```python
from build123d import *

# Parameters (mm, degrees)
ESQUISSE1_W             = 19.5
ESQUISSE1_H             = 1.5
EXTRU_MINCE1_DEPTH      = 127.5
ESQUISSE2_W             = 1.5
ESQUISSE2_H             = 19.5
EXTRU_MINCE2_DEPTH      = 255
ENL_V_MAT_EXTRU_1_DEPTH = 130.132925701
ESQUISSE4_R             = 2.5
ENL_V_MAT_EXTRU_2_DEPTH = 130.409234601
ESQUISSE5_R             = 1.5
ENL_V_MAT_EXTRU_3_DEPTH = 130.350541166
ESQUISSE6_R             = 1.5
ENL_V_MAT_EXTRU_4_DEPTH = 130.409234601


with BuildPart() as part:
    # Esquisse1 → Extru.-Mince1 (new, symmetric)
    with BuildSketch(Plane.XY):
        with Locations((0, 0.75)):
            Rectangle(ESQUISSE1_W, ESQUISSE1_H)
    extrude(amount=EXTRU_MINCE1_DEPTH, both=True)

    # Esquisse2 → Extru.-Mince2 (add)
    with BuildSketch(Plane(origin=(0, 0, -127.5), x_dir=(-1, 0, 0), z_dir=(0, 0, -1))):
        with Locations((0, 9.75)):
            Rectangle(ESQUISSE2_W, ESQUISSE2_H)
    extrude(amount=-EXTRU_MINCE2_DEPTH)

    # Esquisse3 → Enlèv. mat.-Extru.1 (cut, through all)
    with BuildSketch(Plane(origin=(0, 1.5, 0), x_dir=(1, 0, 0), z_dir=(0, 1, 0))):
        with BuildLine():
            Line((-0.75, 127.5), (-0.75, 110))
            ThreePointArc((-0.75, 110), (-8.75, 102), (-16.75, 110))
            Line((-16.75, 110), (-16.75, 127.5))
            ThreePointArc((-16.75, 127.5), (-8.75, 135.5), (-0.75, 127.5))
        make_face()
        with BuildLine():
            Line((17.75, 10), (17.75, -10))
            ThreePointArc((17.75, -10), (9.75, -18), (1.75, -10))
            Line((1.75, -10), (1.75, 10))
            ThreePointArc((1.75, 10), (9.75, 18), (17.75, 10))
        make_face()
        with BuildLine():
            Line((-16.75, -127.5), (-16.75, -110))
            ThreePointArc((-16.75, -110), (-8.75, -102), (-0.75, -110))
            Line((-0.75, -110), (-0.75, -127.5))
            ThreePointArc((-0.75, -127.5), (-8.75, -135.5), (-16.75, -127.5))
        make_face()
    extrude(amount=-ENL_V_MAT_EXTRU_1_DEPTH, mode=Mode.SUBTRACT)

    # Esquisse4 → Enlèv. mat.-Extru.2 (cut, through all)
    with BuildSketch(Plane(origin=(0.75, 0, 0), x_dir=(0, 0, -1), z_dir=(1, 0, 0))):
        with Locations((-120, 10.5)):
            Circle(ESQUISSE4_R)
        with Locations((120, 10.5)):
            Circle(ESQUISSE4_R)
    extrude(amount=-ENL_V_MAT_EXTRU_2_DEPTH, mode=Mode.SUBTRACT)

    # Esquisse5 → Enlèv. mat.-Extru.3 (cut, through all)
    with BuildSketch(Plane.XZ):
        with Locations(Location((-5.75, 59, 0), (0, 0, 270))):
            Circle(ESQUISSE5_R)
        with Locations(Location((-5.75, -59, 0), (0, 0, 90))):
            Circle(ESQUISSE5_R)
    extrude(amount=-ENL_V_MAT_EXTRU_3_DEPTH, mode=Mode.SUBTRACT)

    # Esquisse6 → Enlèv. mat.-Extru.4 (cut, through all)
    with BuildSketch(Plane(origin=(0.75, 0, 0), x_dir=(0, 0, -1), z_dir=(1, 0, 0))):
        with Locations((-51, 6.5)):
            Circle(ESQUISSE6_R)
        with Locations((-15, 6.5)):
            Circle(ESQUISSE6_R)
        with Locations((15, 6.5)):
            Circle(ESQUISSE6_R)
        with Locations((51, 6.5)):
            Circle(ESQUISSE6_R)
    extrude(amount=-ENL_V_MAT_EXTRU_4_DEPTH, mode=Mode.SUBTRACT)


solid = part.part
```
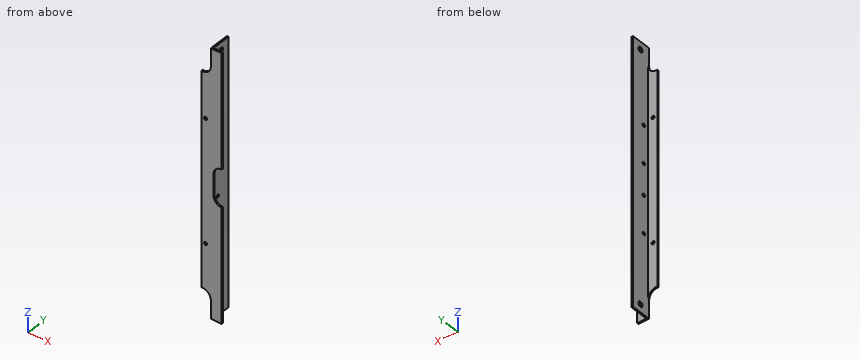
Geometry: final body of the model. Coordinates: model frame, mm. Coordinates: 2 decimals unless noted, no trailing zeros. Order: outer loops, then holes, each group sorted by start corner. A loop starts at its lowest first (then second) coordinate and runs counter-clockwise, first axis right, second up. Notation, with made-up numbers: (38.25, 8.25) - (66.25, 8.25) arc R13 ccw to (66.25, 21.25) - close; hole circle Ø6 at (-25.5, -7). An arc over 180 degrees is marked (long way). Write each question's results on one line, items separated by ' | '.
1) Section C-C, the plane x = 5.25. Return loops of the section in (y, z), plus the area to 3 significant figures.
Results list:
outline: (0, -127.5) - (1.5, -127.5) - (1.5, -16.61) - (0, -16.61) - close; (0, 16.61) - (1.5, 16.61) - (1.5, 127.5) - (0, 127.5) - close | area: 333 mm^2
2) Section D-D, the plane z = -68.5. Return loops of the section in (x, y), plus the area to 4 significant figures.
Results list:
outline: (-9.75, 0) - (9.75, 0) - (9.75, 1.5) - (0.75, 1.5) - (0.75, 19.5) - (-0.75, 19.5) - (-0.75, 1.5) - (-9.75, 1.5) - close | area: 56.25 mm^2
3) Section A-A, the plane z = 120. Return loops of the section in (x, y).
Results list:
outline: (-0.75, 0) - (9.75, 0) - (9.75, 1.5) - (0.75, 1.5) - (0.75, 8) - (-0.75, 8) - close; (-0.75, 13) - (0.75, 13) - (0.75, 19.5) - (-0.75, 19.5) - close
4) Section B-B, the plane y = 10.5. Return loops of the section in (x, z).
Results list:
outline: (-0.75, -127.5) - (0.75, -127.5) - (0.75, -122.5) - (-0.75, -122.5) - close; (-0.75, -117.5) - (0.75, -117.5) - (0.75, 117.5) - (-0.75, 117.5) - close; (-0.75, 122.5) - (0.75, 122.5) - (0.75, 127.5) - (-0.75, 127.5) - close
5) Pin query (flat end, axial travel): pin 1 (4 mm diameter, centred on y = 3, z = 8, fed in from +X); pin 2 (4 mm diameter, centred on y = 6.5, z = 51, fed in from -X); pin 3 (7 mm diameter, centred on x = -5.5, z = 39.5, fed in from +Y). Return the tip coordinate at first contact, or that it passes through.
Results list:
pin 1: x = 1.75 | pin 2: x = -0.75 | pin 3: y = 1.5
6) Line query: line 1 (Y direction, x = 0, z = 120); line 2 (Y direction, x = 0.4, z = -51); line 3 (X direction, y = 7, z = 63). Output: solid intervals per line, ascending. Write a range as from..to.
Results list:
line 1: 0..8, 13..19.5 | line 2: 0..5, 8..19.5 | line 3: -0.75..0.75
